```python
from build123d import *
from build123d.topology import SkipClean

# Parameters (mm, degrees)
BOSS_EXTRUDE1_DEPTH = 4.5
SHELL1_T            = -2.5
SKETCH2_W           = 70.5
SKETCH2_H           = 50.5
CUT_EXTRUDE1_DEPTH  = 6
FILLET1_R           = 2
SKETCH3_R           = 3.25
SKETCH3_R_2         = 1.25
BOSS_EXTRUDE2_DEPTH = 2.5
BOSS_EXTRUDE3_START = 3
BOSS_EXTRUDE3_DEPTH = 3
SKETCH5_W           = 12.567423642
SKETCH5_H           = 1.646842997
BOSS_EXTRUDE4_DEPTH = 4
BOSS_EXTRUDE5_DEPTH = 12.567423642
FILLET4_R           = 3
SKETCH8_W           = 70.5
SKETCH8_H           = 50.5
CUT_EXTRUDE2_DEPTH  = 4
BOSS_EXTRUDE6_START = 4
BOSS_EXTRUDE6_DEPTH = 4
CHAMFER1_SIZE       = 1.25
SKETCH11_W          = 15.487290784
SKETCH11_H          = 50.5
CUT_EXTRUDE3_DEPTH  = 24
CUT_EXTRUDE4_START  = -6.5
SKETCH13_R          = 3.25
CUT_EXTRUDE4_DEPTH  = 6.5
SKETCH14_R          = 0.75
BOSS_EXTRUDE7_DEPTH = 0.5
FILLET5_R           = 0.5
BOSS_EXTRUDE8_START = 0.5
SKETCH15_R          = 0.75
BOSS_EXTRUDE8_DEPTH = 0.5
FILLET6_R           = 0.5
SKETCH16_W          = 32.358974192
SKETCH16_H          = 1.7505668
CUT_EXTRUDE5_DEPTH  = 20.5
SKETCH17_R          = 0.783892082
CUT_EXTRUDE6_DEPTH  = 78.755475754


# Some blends are built 0.0001 mm under size
with BuildPart() as part:
    # Sketch1 → Boss-Extrude1 (new body)
    with BuildSketch(Plane(origin=(0, 0, 0), x_dir=(1, 0, 0), z_dir=(0, 1, 0))):
        with BuildLine():
            Line((46.356686108, -24.641010635), (46.356686108, 24.641010635))
            ThreePointArc((46.356686108, 24.641010635), (44.306433576, 29.590758103), (39.356686108, 31.641010635))
            Line((39.356686108, 31.641010635), (-39.356686108, 31.641010635))
            ThreePointArc((-39.356686108, 31.641010635), (-44.306433576, 29.590758103), (-46.356686108, 24.641010635))
            Line((-46.356686108, 24.641010635), (-46.356686108, -24.641010635))
            ThreePointArc((-46.356686108, -24.641010635), (-44.306433576, -29.590758103), (-39.356686108, -31.641010635))
            Line((-39.356686108, -31.641010635), (39.356686108, -31.641010635))
            ThreePointArc((39.356686108, -31.641010635), (44.306433576, -29.590758103), (46.356686108, -24.641010635))
        make_face()
    extrude(amount=BOSS_EXTRUDE1_DEPTH)

    # Shell1
    shell1_openings = [part.faces().sort_by_distance(p)[0] for p in [
        (0, 0, 0),
    ]]
    offset(amount=SHELL1_T, openings=shell1_openings, kind=Kind.INTERSECTION)

    # Sketch2 → Cut-Extrude1 (cut)
    with BuildSketch(Plane(origin=(0, 4.5, 0), x_dir=(1, 0, 0), z_dir=(0, 1, 0))):
        with Locations((0.393313892, -1.108989365)):
            Rectangle(SKETCH2_W, SKETCH2_H)
    extrude(amount=-CUT_EXTRUDE1_DEPTH, mode=Mode.SUBTRACT)

    # Fillet1
    fillet1_edges = [part.edges().sort_by_distance(p)[0] for p in [
        (42.538666623, 2, 27.82299115),
        (0, 2, 29.141010635),
        (-42.538666623, 2, 27.82299115),
        (-43.856686108, 2, 0),
        (-42.538666623, 2, -27.82299115),
        (0, 2, -29.141010635),
        (42.538666623, 2, -27.82299115),
        (43.856686108, 2, 0),
    ]]
    fillet(fillet1_edges, radius=FILLET1_R - 0.0001)  # a hair under: the kernel refuses the full size

    # Sketch3 → Boss-Extrude2 (add)
    # profile 1 of 4: a face of its own
    with BuildSketch(Plane.XZ.offset(-2)):
        with Locations(Location((-40.393075335, 23.335972527, 0), (0, 0, 100.663495608))):
            Circle(SKETCH3_R)
        with Locations(Location((-40.393075335, 23.335972527, 0), (0, 0, 270))):
            Circle(SKETCH3_R_2, mode=Mode.SUBTRACT)
    # profile 2 of 4: a face of its own
    with BuildSketch(Plane.XZ.offset(-2)):
        with Locations(Location((-40.393075335, -25.664027473, 0), (0, 0, 116.76561408))):
            Circle(SKETCH3_R)
        with Locations(Location((-40.393075335, -25.664027473, 0), (0, 0, 179.461771678))):
            Circle(SKETCH3_R_2, mode=Mode.SUBTRACT)
    # profile 3 of 4: a face of its own
    with BuildSketch(Plane.XZ.offset(-2)):
        with Locations(Location((37.638494393, -25.664027473, 0), (0, 0, 127.872158601))):
            Circle(SKETCH3_R)
        with Locations(Location((37.638494393, -25.664027473, 0), (0, 0, 270))):
            Circle(SKETCH3_R_2, mode=Mode.SUBTRACT)
    # profile 4 of 4: a face of its own
    with BuildSketch(Plane.XZ.offset(-2)):
        with Locations(Location((37.638494393, 23.335972526, 0), (0, 0, 127.872158601))):
            Circle(SKETCH3_R)
        with Locations(Location((37.638494393, 23.335972526, 0), (0, 0, 270))):
            Circle(SKETCH3_R_2, mode=Mode.SUBTRACT)
    extrude(amount=BOSS_EXTRUDE2_DEPTH)

    # Sketch4 → Boss-Extrude3 (add)
    with SkipClean():  # the faces are left unmerged after this step: merging them gives an invalid solid
        with BuildSketch(Plane.XZ.offset(BOSS_EXTRUDE3_START)):
            with BuildLine():
                Line((39.356686108, 31.641010635), (-39.356686108, 31.641010635))
                ThreePointArc((-39.356686108, 31.641010635), (-44.306433576, 29.590758103), (-46.356686108, 24.641010635))
                Line((-46.356686108, 24.641010635), (-46.356686108, -24.641010635))
                ThreePointArc((-46.356686108, -24.641010635), (-44.306433576, -29.590758103), (-39.356686108, -31.641010635))
                Line((-39.356686108, -31.641010635), (39.356686108, -31.641010635))
                ThreePointArc((39.356686108, -31.641010635), (44.306433576, -29.590758103), (46.356686108, -24.641010635))
                Line((46.356686108, -24.641010635), (46.356686108, 24.641010635))
                ThreePointArc((46.356686108, 24.641010635), (44.306433576, 29.590758103), (39.356686108, 31.641010635))
            make_face()
            with BuildLine():
                Line((39.356686108, 29.141010635), (-39.356686108, 29.141010635))
                ThreePointArc((-39.356686108, 29.141010635), (-42.538666623, 27.82299115), (-43.856686108, 24.641010635))
                Line((-43.856686108, 24.641010635), (-43.856686108, -24.641010635))
                ThreePointArc((-43.856686108, -24.641010635), (-42.538666623, -27.82299115), (-39.356686108, -29.141010635))
                Line((-39.356686108, -29.141010635), (39.356686108, -29.141010635))
                ThreePointArc((39.356686108, -29.141010635), (42.538666623, -27.82299115), (43.856686108, -24.641010635))
                Line((43.856686108, -24.641010635), (43.856686108, 24.641010635))
                ThreePointArc((43.856686108, 24.641010635), (42.538666623, 27.82299115), (39.356686108, 29.141010635))
            make_face(mode=Mode.SUBTRACT)
        extrude(amount=-BOSS_EXTRUDE3_DEPTH)

    # Sketch5 → Boss-Extrude4 (add)
    with SkipClean():  # the faces are left unmerged after this step: merging them gives an invalid solid
        with BuildSketch(Plane(origin=(-34.856686108, 0, 0), x_dir=(0, 0, -1), z_dir=(1, 0, 0))):
            with Locations((0.008961538, 1.176578502)):
                Rectangle(SKETCH5_W, SKETCH5_H)
        extrude(amount=-BOSS_EXTRUDE4_DEPTH)

    # Sketch6 → Boss-Extrude5 (add)
    with SkipClean():  # the faces are left unmerged after this step: merging them gives an invalid solid
        with BuildSketch(Plane.XY.offset(6.274750283)):
            Polygon((-34.856686108, 0.353157003), (-32.884887287, 0.353157003), (-32.884887287, -0.785578936), (-38.308352122, -0.785578936), (-38.856686108, 0.353157003), align=None)
        extrude(amount=-BOSS_EXTRUDE5_DEPTH)

    # Fillet4
    # the kernel refuses this fillet: 3 mm, written as the material it takes off along each edge
    with BuildSketch(Plane(origin=(-32.884887287, 7.853157003, -6.292673359), x_dir=(-1, 0, 0), z_dir=(0, -1, 0))) as fillet4_piece_1_section:
        with BuildLine():
            CenterArc((FILLET4_R, -FILLET4_R), FILLET4_R, 90, 90)
            Line((0, -FILLET4_R), (0, 0))
            Line((0, 0), (FILLET4_R, 0))
        make_face()
    fillet4_piece_1 = extrude(amount=16.138735939, mode=Mode.PRIVATE)
    fillet4_piece_1 = split(fillet4_piece_1, bisect_by=Plane(origin=(-35.112153747, 2, -6.238457851), z_dir=(0, -1, 0)), keep=Keep.TOP, mode=Mode.PRIVATE)
    add(fillet4_piece_1, mode=Mode.SUBTRACT)
    with BuildSketch(Plane(origin=(-32.884887287, 7.853157003, 6.274750283), x_dir=(-1, 0, 0), z_dir=(0, -1, 0))) as fillet4_piece_2_section:
        with BuildLine():
            CenterArc((FILLET4_R, FILLET4_R), FILLET4_R, 180, 90)
            Line((0, FILLET4_R), (0, 0))
            Line((0, 0), (FILLET4_R, 0))
        make_face()
    fillet4_piece_2 = extrude(amount=16.138735939, mode=Mode.PRIVATE)
    fillet4_piece_2 = split(fillet4_piece_2, bisect_by=Plane(origin=(-35.112153747, 2, 6.220534774), z_dir=(0, -1, 0)), keep=Keep.TOP, mode=Mode.PRIVATE)
    add(fillet4_piece_2, mode=Mode.SUBTRACT)

    # Sketch8 → Cut-Extrude2 (cut)
    with BuildSketch(Plane(origin=(0, 4.5, 0), x_dir=(1, 0, 0), z_dir=(0, 1, 0))):
        with Locations((0.393313892, -1.108989365)):
            Rectangle(SKETCH8_W, SKETCH8_H)
    extrude(amount=-CUT_EXTRUDE2_DEPTH, mode=Mode.SUBTRACT)

    # Sketch10 → Boss-Extrude6 (add)
    with BuildSketch(Plane.XZ.offset(3).offset(BOSS_EXTRUDE6_START)):
        with BuildLine():
            Line((-39.356686108, -30.391010635), (39.356686108, -30.391010635))
            ThreePointArc((39.356686108, -30.391010635), (43.4225501, -28.706874627), (45.106686108, -24.641010635))
            Line((45.106686108, -24.641010635), (45.106686108, 24.641010635))
            ThreePointArc((45.106686108, 24.641010635), (43.4225501, 28.706874627), (39.356686108, 30.391010635))
            Line((39.356686108, 30.391010635), (-39.356686108, 30.391010635))
            ThreePointArc((-39.356686108, 30.391010635), (-43.4225501, 28.706874627), (-45.106686108, 24.641010635))
            Line((-45.106686108, 24.641010635), (-45.106686108, -24.641010635))
            ThreePointArc((-45.106686108, -24.641010635), (-43.4225501, -28.706874627), (-39.356686108, -30.391010635))
        make_face()
        with BuildLine():
            Line((-39.356686108, -29.141010635), (39.356686108, -29.141010635))
            ThreePointArc((39.356686108, -29.141010635), (42.538666623, -27.82299115), (43.856686108, -24.641010635))
            Line((43.856686108, -24.641010635), (43.856686108, 24.641010635))
            ThreePointArc((43.856686108, 24.641010635), (42.538666623, 27.82299115), (39.356686108, 29.141010635))
            Line((39.356686108, 29.141010635), (-39.356686108, 29.141010635))
            ThreePointArc((-39.356686108, 29.141010635), (-42.538666623, 27.82299115), (-43.856686108, 24.641010635))
            Line((-43.856686108, 24.641010635), (-43.856686108, -24.641010635))
            ThreePointArc((-43.856686108, -24.641010635), (-42.538666623, -27.82299115), (-39.356686108, -29.141010635))
        make_face(mode=Mode.SUBTRACT)
    extrude(amount=-BOSS_EXTRUDE6_DEPTH)

    # Chamfer1
    chamfer1_edges = [part.edges().sort_by_distance(p)[0] for p in [
        (-43.4225501, -3, -28.706874627),
        (0, -3, -30.391010635),
        (43.4225501, -3, -28.706874627),
        (45.106686108, -3, 0),
        (43.4225501, -3, 28.706874627),
        (0, -3, 30.391010635),
        (-43.4225501, -3, 28.706874627),
        (-45.106686108, -3, 0),
    ]]
    chamfer(chamfer1_edges, length=CHAMFER1_SIZE - 0.0001)  # a hair under: the kernel refuses the full size

    # Sketch11 → Cut-Extrude3 (cut)
    with BuildSketch(Plane(origin=(0, 4.5, 0), x_dir=(1, 0, 0), z_dir=(0, 1, 0))):
        with Locations((27.8996685, -1.108989365)):
            Rectangle(SKETCH11_W, SKETCH11_H)
    extrude(amount=-CUT_EXTRUDE3_DEPTH, mode=Mode.SUBTRACT)

    # Sketch13 → Cut-Extrude4 (cut)
    with BuildSketch(Plane.XZ.offset(7).offset(CUT_EXTRUDE4_START)):
        with Locations((-40.393075335, -25.664027473)):
            Circle(SKETCH13_R)
    extrude(amount=CUT_EXTRUDE4_DEPTH, mode=Mode.SUBTRACT)

    # Sketch14 → Boss-Extrude7 (add)
    with BuildSketch(Plane(origin=(0, 0, -30.391010635), x_dir=(-1, 0, 0), z_dir=(0, 0, -1))):
        with Locations(Location((0, -5.25, 0), (0, 0, 180))):
            Circle(SKETCH14_R)
    extrude(amount=BOSS_EXTRUDE7_DEPTH)

    # Fillet5
    fillet5_edges = [part.edges().sort_by_distance(p)[0] for p in [
        (-0.75, -5.25, -30.891010635),
    ]]
    fillet(fillet5_edges, radius=FILLET5_R - 0.0001)  # a hair under: the kernel refuses the full size

    # Sketch15 → Boss-Extrude8 (add)
    with BuildSketch(Plane.XY.offset(30.391010635).offset(BOSS_EXTRUDE8_START)):
        with Locations(Location((0, -5.25, 0), (0, 0, 180))):
            Circle(SKETCH15_R)
    extrude(amount=-BOSS_EXTRUDE8_DEPTH)

    # Fillet6
    fillet6_edges = [part.edges().sort_by_distance(p)[0] for p in [
        (0.75, -5.25, 30.891010635),
    ]]
    fillet(fillet6_edges, radius=FILLET6_R - 0.0001)  # a hair under: the kernel refuses the full size

    # Sketch16 → Cut-Extrude5 (cut)
    with BuildSketch(Plane(origin=(45.106686108, 0, 0), x_dir=(0, 0, -1), z_dir=(1, 0, 0))):
        with Locations((11.286987709, -6.446354596)):
            Rectangle(SKETCH16_W, SKETCH16_H)
    extrude(amount=-CUT_EXTRUDE5_DEPTH, mode=Mode.SUBTRACT)

    # Sketch17 → Cut-Extrude6 (cut, through all)
    with BuildSketch(Plane(origin=(0, 0, -30.391010635), x_dir=(-1, 0, 0), z_dir=(0, 0, -1))):
        with Locations((23.679650241, -5.268916998)):
            Circle(SKETCH17_R)
        with Locations((-23.679650241, -5.268916998)):
            Circle(SKETCH17_R)
    extrude(amount=-CUT_EXTRUDE6_DEPTH, mode=Mode.SUBTRACT)


solid = part.part
```
Work out the finished part from the listing and answer in its coordinate system (mm). A direction names the side the tool comes from. Coordinates: 2 decimals unless noted, no trailing zeros.
1) Consider probe 1 along X at (y, z) = (0, -11); probe 2 along Z at (x, y) = (31, -1); probe 3 along Z at (x, y) = (-4.5, 3.5). Determine where each line is inside the solid, lowest interval first.
Results:
probe 1: x = -46.36 to -43.86, 43.86 to 46.36
probe 2: z = -31.64 to -29.14, 29.14 to 31.64
probe 3: z = -31.64 to -24.14, 26.36 to 31.64
2) Flat-ended cylindrical pins translate along their axes: pin 1 (4 mm diameter, centred on x = -40.39, z = 23.34, fed in from -Y); pin 2 (1.6 mm diameter, centred on x = -35.5, z = 2.5, fed in from -Y); pin 3 (1.5 mm diameter, centred on x = 36, z = 10, fed in from -Y). Find the tip coordinate at first contact, or state that the pin passes through.
Results:
pin 1: stops at y = -0.5
pin 2: stops at y = -0.79
pin 3: stops at y = 2
3) For faces 1 (the flat face through (-34.857, 3, 1)), 2 (the flat face through (1, -4, 29.141)), 3 (the cylindrical face through (42.6, -5.64, -29.39)), 4 (the flat face through (46.357, 1, 0)), 5 (the flat face through (0, 3, 26.359)), determine the directions among +Z, -Z, +X, -X, +Y, -Y from which every point of the face is accessible in a straight line to the end or side of a thin tool.
Results:
face 1: +Y
face 2: -Y
face 3: -Z, +X, -Y
face 4: +Z, -Z, +X, +Y, -Y
face 5: +Y, -Y
4) For a pull along Z with two mould halves and no side action, classify faces 6 (the flat face through (-1, 4.5, 28)), 7 (the conical face through (-43.614, -3.911, 28.993)), 8 (the cylindrical face through (44.361, 0.697, -29.536)), 9 (the flat face through (0, 3, -24.141)) as +Z half, -Z half, draft (parallel to the pull), parting line (faces both ways), or undercut.
Results:
face 6: draft
face 7: +Z half
face 8: -Z half
face 9: undercut
